from build123d import *

# Parameters (mm, degrees)
SKETCH1_W           = 64
SKETCH1_H           = 82
SKETCH1_R           = 1.75
SKETCH1_W_2         = 28
SKETCH1_H_2         = 36
BOSS_EXTRUDE1_DEPTH = 2
SKETCH4_W           = 4
SKETCH4_H           = 4
SKETCH4_H_2         = 7
BOSS_EXTRUDE2_DEPTH = 10
CUT_EXTRUDE1_DEPTH  = 3
DRAFT12_ANGLE       = 10
DRAFT13_ANGLE       = 10
SKETCH6_W           = 18.473460386
SKETCH6_H           = 9
CUT_EXTRUDE2_DEPTH  = 3
FILLET1_R           = 3
FILLET2_R           = 3


with BuildPart() as part:
    # Sketch1 → Boss-Extrude1 (new body)
    with BuildSketch(Plane(origin=(0, 0, 0), x_dir=(1, 0, 0), z_dir=(0, 1, 0))):
        Rectangle(SKETCH1_W, SKETCH1_H)
        with Locations((27.75, -36.6)):
            Circle(SKETCH1_R, mode=Mode.SUBTRACT)
        with Locations((-27.75, -36.6)):
            Circle(SKETCH1_R, mode=Mode.SUBTRACT)
        with Locations((-27.75, 36.6)):
            Circle(SKETCH1_R, mode=Mode.SUBTRACT)
        with Locations((27.75, 36.6)):
            Circle(SKETCH1_R, mode=Mode.SUBTRACT)
        Rectangle(SKETCH1_W_2, SKETCH1_H_2, mode=Mode.SUBTRACT)
    extrude(amount=BOSS_EXTRUDE1_DEPTH)

    # Sketch4 → Boss-Extrude2 (add)
    with BuildSketch(Plane(origin=(0, 2, 0), x_dir=(1, 0, 0), z_dir=(0, 1, 0))):
        with Locations((-17, -25)):
            Rectangle(SKETCH4_W, SKETCH4_H)
        with Locations((17, -25)):
            Rectangle(SKETCH4_W, SKETCH4_H)
        with Locations((-17, 25)):
            Rectangle(SKETCH4_W, SKETCH4_H)
        with Locations((17, 25)):
            Rectangle(SKETCH4_W, SKETCH4_H)
        with Locations((-22, -17.5)):
            Rectangle(SKETCH4_W, SKETCH4_H_2)
        with Locations((22, -17.5)):
            Rectangle(SKETCH4_W, SKETCH4_H_2)
        with Locations((-22, 19)):
            Rectangle(SKETCH4_W, SKETCH4_H)
        with Locations((22, 19)):
            Rectangle(SKETCH4_W, SKETCH4_H)
    extrude(amount=BOSS_EXTRUDE2_DEPTH)

    # Sketch5 → Cut-Extrude1 (cut, through all)
    with BuildSketch(Plane(origin=(0, 2, 0), x_dir=(1, 0, 0), z_dir=(0, 1, 0))):
        Polygon((-32, 32), (-24, 21), (-24, -21), (-32, -32), align=None)
        Polygon((32, -32), (24, -21), (24, 21), (32, 32), align=None)
    extrude(amount=-CUT_EXTRUDE1_DEPTH, mode=Mode.SUBTRACT)

    # Draft12
    draft12_faces = [part.faces().sort_by_distance(p)[0] for p in [
        (22, 7, 14),
        (22, 7, -17),
        (-22, 7, 14),
        (-22, 7, -17),
    ]]
    draft(draft12_faces, Plane.ZX.offset(12), DRAFT12_ANGLE)

    # Draft13
    draft13_faces = [part.faces().sort_by_distance(p)[0] for p in [
        (15, 7, 25),
        (-15, 7, 25),
        (15, 7, -25),
        (-15, 7, -25),
    ]]
    draft(draft13_faces, Plane.ZX.offset(12), DRAFT13_ANGLE)

    # Sketch6 → Cut-Extrude2 (cut, through all)
    with BuildSketch(Plane(origin=(0, 2, 0), x_dir=(1, 0, 0), z_dir=(0, 1, 0))):
        Polygon((-22, 41), (-17.636363636, 35), (17.636363636, 35), (22, 41), align=None)
        with BuildLine():
            Line((17, 10), (17, -6))
            ThreePointArc((17, -6), (19, -8), (21, -6))
            Line((21, -6), (21, 10))
            ThreePointArc((21, 10), (19, 12), (17, 10))
        make_face()
        Polygon((22, -41), (17.636363636, -35), (-17.636363636, -35), (-22, -41), align=None)
        with Locations((0, 26.5)):
            Rectangle(SKETCH6_W, SKETCH6_H)
        with Locations((0, -26.5)):
            Rectangle(SKETCH6_W, SKETCH6_H)
        with BuildLine():
            Line((-17, 10), (-17, -6))
            ThreePointArc((-17, -6), (-19, -8), (-21, -6))
            Line((-21, -6), (-21, 10))
            ThreePointArc((-21, 10), (-19, 12), (-17, 10))
        make_face()
    extrude(amount=-CUT_EXTRUDE2_DEPTH, mode=Mode.SUBTRACT)

    # Fillet1
    fillet1_edges = [part.edges().sort_by_distance(p)[0] for p in [
        (-32, 1, 32),
        (-32, 1, -32),
        (32, 1, -32),
        (32, 1, 32),
        (-22, 1, -41),
        (22, 1, -41),
        (22, 1, 41),
        (-22, 1, 41),
        (32, 1, 41),
        (-32, 1, 41),
        (-32, 1, -41),
        (32, 1, -41),
    ]]
    fillet(fillet1_edges, radius=FILLET1_R)

    # Fillet2
    fillet2_edges = [part.edges().sort_by_distance(p)[0] for p in [
        (-22, 2, 12.236730193),
        (22, 2, -15.236730193),
        (-22, 2, -15.236730193),
        (13.236730193, 2, 25),
        (-13.236730193, 2, 25),
        (-13.236730193, 2, -25),
        (13.236730193, 2, -25),
        (22, 2, 12.236730193),
    ]]
    fillet(fillet2_edges, radius=FILLET2_R)


solid = part.part
The model under review builds one solid part; all positions refer to its coordinate system, in mm. A direction names the side the tool comes from. Give positions to 0.01 mm unless a question says otherwise; leave off trailing zeros. Order: outer loops, then holes, each group sorted by start corner. A loop starts at its lowest first (then second) coordinate and runs counter-clockwise, first axis right, second up. Notation, with made-up numbers: M 30,3 L 47,3 A7 ccw 47,14 Z; hole C 26,83 d8. An arc over 180 degrees is marked long. Answer in a Markdown table with one row per item. Add a question column.
1. For pin 1 Ø1.6 at (y, z) = (1, -26) entering from +X; pin 2 Ø3 at (y, z) = (9.5, -25) entering from +X; pin 3 Ø2 at (x, y) = (-4.5, 1.5) entering from +Z, all flat-tipped, find the tip position at first contact; note any pin that passes through.
2. Add section B-B on z = 15. State the section outline as (x, y) points.
3. Machinability: for faces 5 (the flat face through (9.237, 1, -26)), 6 (the flat face through (24, 1, 5)), 7 (the flat face through (-24, 1, 4)), 8 (the flat face through (-22, 7, 21)), 9 (the flat face through (-17, 7, 23)), which of the approach directions +Z, -Z, +X, -X, +Y, -Y give a long, thin tool a straight path to every point of the face, cutting with its end or side? Answer none if there is none.
4. Add section D-D on y = 9.25. Count the separate pieces of the cut face and the enclosed holes in it, plus the area to 3 significant figures.
5. Mouldability with a two-part tool opening along X and no side actions: class faces 1 (the cylindrical face through (-29.5, 0.99, 36.52)), 2 (the flat face through (-14, 1, 0)), 3 (the flat face through (32, 1, 36)), 4 (the flat face through (17, 7, -23)) as released by +X, released by -X, zero draft, split by the parting line, or undercut.
6. Add section A-A on z = -8. State the section outline as (x, y) points.
7. To check wall thickness, follow line 1 along X through (y, z) = (6, -18); line 2 along Z through (x, y) = (27.75, 0.9); line 3 along X through (y, z) = (0.7, 36.6). State the ranges of each line that lie inside material, in increasing order.
8. Add section C-C on x = -3. State the section outline as (y, z) points, plus the area to 3 significant figures.
The answers:
| question | item | result |
|---|---|---|
| 1 | pin 1 | x = 28.22 |
| 1 | pin 2 | x = 19 |
| 1 | pin 3 | z = 35 |
| 2 | outline | M -24,0 L -14,0 L -14,2 L -20,2 L -20,12 L -24,12 Z; M 14,0 L 24,0 L 24,12 L 20,12 L 20,2 L 14,2 Z |
| 3 | face 5 | +Y, -Y |
| 3 | face 6 | +X, +Y, -Y |
| 3 | face 7 | -X, +Y, -Y |
| 3 | face 8 | +Z, +X, -X, +Y |
| 3 | face 9 | +X, -X, +Y |
| 4 | separate pieces | 8 |
| 4 | enclosed holes | 0 |
| 4 | area | 168 mm2 |
| 5 | face 1 | undercut |
| 5 | face 2 | undercut |
| 5 | face 3 | released by +X |
| 5 | face 4 | zero draft |
| 6 | outline | M -24,0 L -21,0 L -21,2 L -24,2 Z; M -17,0 L -14,0 L -14,2 L -17,2 Z; M 14,0 L 17,0 L 17,2 L 14,2 Z; M 21,0 L 24,0 L 24,2 L 21,2 Z |
| 7 | line 1 | -24 to -20, 20 to 24 |
| 7 | line 2 | -41 to -38.35, -34.85 to -26.16, 26.16 to 34.85, 38.35 to 41 |
| 7 | line 3 | -32 to -29.5, -26 to -18.8, 18.8 to 26, 29.5 to 32 |
| 8 | outline | M 0,-35 L 2,-35 L 2,-31 L 0,-31 Z; M 0,-22 L 2,-22 L 2,-18 L 0,-18 Z; M 0,18 L 2,18 L 2,22 L 0,22 Z; M 0,31 L 2,31 L 2,35 L 0,35 Z |
| 8 | area | 32.0 mm2 |
